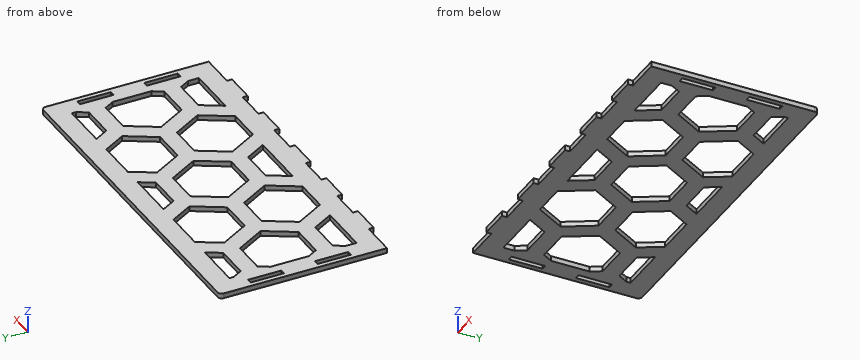
from build123d import *

# Parameters (mm, degrees)
SKETCH1_W               = 3.05
SKETCH1_H               = 20
SKETCH1_W_2             = 18.272727272
SKETCH1_H_2             = 3
SKETCH1_W_3             = 18.272727273
BOSS_EXTRUDE1_DEPTH     = 3
SKETCH5_W               = 207
SKETCH5_H               = 40
CUT_EXTRUDE7_DEPTH      = 1
CUT_EXTRUDE7_DEPTH_BACK = 4
FILLET3_R               = 2.5
CUT_EXTRUDE8_DEPTH      = 4
CUT_EXTRUDE8_DEPTH_BACK = 1


with BuildPart() as part:
    # Sketch1 → Boss-Extrude1 (new body)
    with BuildSketch(Plane.XY):
        Polygon((-103.5, 70), (-103.5, -70), (-82.227272727, -70), (-63.954545455, -70), (-45.681818182, -70), (-27.409090909, -70), (-9.136363636, -70), (9.136363636, -70), (27.409090909, -70), (45.681818182, -70), (63.954545455, -70), (82.227272727, -70), (103.5, -70), (103.5, 70), align=None)
        with Locations((-98.975, -40)):
            Rectangle(SKETCH1_W, SKETCH1_H, mode=Mode.SUBTRACT)
        with Locations((98.975, -40)):
            Rectangle(SKETCH1_W, SKETCH1_H, mode=Mode.SUBTRACT)
        with Locations((-98.975, 0)):
            Rectangle(SKETCH1_W, SKETCH1_H, mode=Mode.SUBTRACT)
        with Locations((-98.975, 40)):
            Rectangle(SKETCH1_W, SKETCH1_H, mode=Mode.SUBTRACT)
        with Locations((98.975, 0)):
            Rectangle(SKETCH1_W, SKETCH1_H, mode=Mode.SUBTRACT)
        with Locations((98.975, 40)):
            Rectangle(SKETCH1_W, SKETCH1_H, mode=Mode.SUBTRACT)
        with Locations((-73.090909091, -71.5)):
            Rectangle(SKETCH1_W_2, SKETCH1_H_2)
        with Locations((-36.545454546, -71.5)):
            Rectangle(SKETCH1_W_3, SKETCH1_H_2)
        with Locations((0, -71.5)):
            Rectangle(SKETCH1_W_2, SKETCH1_H_2)
        with Locations((36.545454546, -71.5)):
            Rectangle(SKETCH1_W_3, SKETCH1_H_2)
        with Locations((73.090909091, -71.5)):
            Rectangle(SKETCH1_W_2, SKETCH1_H_2)
    extrude(amount=BOSS_EXTRUDE1_DEPTH)

    # Sketch5 → Cut-Extrude7 (cut, two sides)
    with BuildSketch(Plane.XY.offset(3)) as cut_extrude7_sk:
        with Locations((0, 50)):
            Rectangle(SKETCH5_W, SKETCH5_H)
    extrude(amount=CUT_EXTRUDE7_DEPTH, mode=Mode.SUBTRACT)
    extrude(cut_extrude7_sk.sketch, amount=-CUT_EXTRUDE7_DEPTH_BACK, mode=Mode.SUBTRACT)

    # Fillet3
    fillet3_edges = [part.edges().sort_by_distance(p)[0] for p in [
        (103.5, 30, 1.5),
        (-103.5, 30, 1.5),
    ]]
    fillet(fillet3_edges, radius=FILLET3_R)

    # Sketch6 → Cut-Extrude8 (cut, two sides)
    with BuildSketch(Plane.XY) as cut_extrude8_sk:
        Polygon((-88.045916051, -0.5), (-91.5, -6.482648893), (-91.5, -29.517351107), (-88.045916051, -35.5), (-67.83865663, -35.5), (-57.735026919, -18), (-67.83865663, -0.5), align=None)
        Polygon((-62.931179342, 18), (-91.5, 18), (-91.5, 15.482648893), (-88.045916051, 9.5), (-67.83865663, 9.5), align=None)
        Polygon((-26.558112383, 18), (-51.384173958, 18), (-59.178402592, 4.5), (-49.074772881, -13), (-28.867513459, -13), (-18.763883749, 4.5), align=None)
        Polygon((10.103629711, -35.5), (20.207259422, -18), (10.103629711, -0.5), (-10.103629711, -0.5), (-20.207259422, -18), (-10.103629711, -35.5), align=None)
        Polygon((51.384173958, 18), (26.558112383, 18), (18.763883749, 4.5), (28.867513459, -13), (49.074772881, -13), (59.178402592, 4.5), align=None)
        Polygon((91.5, -29.517351107), (91.5, -6.482648893), (88.045916051, -0.5), (67.83865663, -0.5), (57.735026919, -18), (67.83865663, -35.5), (88.045916051, -35.5), align=None)
        Polygon((91.5, 15.482648893), (91.5, 18), (62.931179342, 18), (67.83865663, 9.5), (88.045916051, 9.5), align=None)
        Polygon((15.011106999, 18), (-15.011106999, 18), (-10.103629711, 9.5), (10.103629711, 9.5), align=None)
        Polygon((-28.867513459, -23), (-49.074772881, -23), (-59.178402592, -40.5), (-49.074772881, -58), (-28.867513459, -58), (-18.763883749, -40.5), align=None)
        Polygon((-88.045916051, -45.5), (-91.5, -51.482648893), (-91.5, -58), (-60.621778265, -58), (-67.83865663, -45.5), align=None)
        Polygon((-10.103629711, -45.5), (-17.320508076, -58), (17.320508076, -58), (10.103629711, -45.5), align=None)
        Polygon((49.074772881, -23), (28.867513459, -23), (18.763883749, -40.5), (28.867513459, -58), (49.074772881, -58), (59.178402592, -40.5), align=None)
        Polygon((91.5, -58), (91.5, -51.482648893), (88.045916051, -45.5), (67.83865663, -45.5), (60.621778265, -58), align=None)
    extrude(amount=CUT_EXTRUDE8_DEPTH, mode=Mode.SUBTRACT)
    extrude(cut_extrude8_sk.sketch, amount=-CUT_EXTRUDE8_DEPTH_BACK, mode=Mode.SUBTRACT)


solid = part.part
The listing builds one solid part. Answer for the finished solid, in the listing's coordinates (mm). Round coordinates to 2 decimals unless told otherwise and drop trailing zeros. Loops run counter-clockwise (first coordinate to the right, second up) from the corner with the lowest first, then second, coordinate; pieces in that order, holes last. Notation, with made-up numbers: M 82.5,85 L 136.5,85 A25 cw 136.5,106 Z; hole C 83,27 d1. An arc over 180 degrees is marked long. Return JSON: item names as keys, results as strings.
Q1. Find section A-A, the plane x = -86. Determine the outline of the cut face in (y, z).
Results list:
{"outline": "M -70,0 L -58,0 L -58,3 L -70,3 Z; M -45.5,0 L -35.5,0 L -35.5,3 L -45.5,3 Z; M -0.5,0 L 9.5,0 L 9.5,3 L -0.5,3 Z; M 18,0 L 30,0 L 30,3 L 18,3 Z"}
Q2. Find section C-C, the plane y = -20. Determine the outline of the cut face in (x, z).
Results list:
{"outline": "M -103.5,0 L -91.5,0 L -91.5,3 L -103.5,3 Z; M -58.89,0 L -19.05,0 L -19.05,3 L -58.89,3 Z; M 19.05,0 L 58.89,0 L 58.89,3 L 19.05,3 Z; M 91.5,0 L 103.5,0 L 103.5,3 L 91.5,3 Z"}
Q3. Find the intervals of material crossed by line 1 along Y through (x, z) = (-2, 0.7); line 2 along Y through (x, z) = (47, 1.25); line 3 along Y through (x, z) = (-86, 0.6), in increasing order. Write a range as from..to.
Results list:
{"line 1": "y = -73..-58, -45.5..-35.5, -0.5..9.5, 18..30", "line 2": "y = -70..-58, -23..-13, 18..30", "line 3": "y = -70..-58, -45.5..-35.5, -0.5..9.5, 18..30"}
Q4. Find section D-D, the plane z = 1.95. State how many separate pieces and enclosed holes the cut face has, plus the area to 3 significant figures.
Results list:
{"separate pieces": "1", "enclosed holes": "17", "area": "12,000 mm2"}
Q5. This flat-tipped pin is pushed along its axis until it touches: pin 1 Ø0.9 at (x, z) = (-98.5, 1) entering from -Y. Where does it stop, or does it pass through?
Results list:
{"pin 1": "stops at y = -70"}
Q6. Find section B-B, the plane y = -43. Determine the outline of the cut face in (x, z).
Results list:
{"outline": "M -103.5,0 L -100.5,0 L -100.5,3 L -103.5,3 Z; M -97.45,0 L -57.74,0 L -57.74,3 L -97.45,3 Z; M -20.21,0 L 20.21,0 L 20.21,3 L -20.21,3 Z; M 57.74,0 L 97.45,0 L 97.45,3 L 57.74,3 Z; M 100.5,0 L 103.5,0 L 103.5,3 L 100.5,3 Z"}
